```python
from build123d import *

# Parameters (mm, degrees)
SKETCH2_R               = 31.5
SKETCH2_R_2             = 4.5
BOSS_EXTRUDE2_DEPTH     = 20
CUT_EXTRUDE1_DEPTH      = 26
CUT_EXTRUDE1_DEPTH_BACK = 80
SKETCH3_W               = 10.2
SKETCH3_H               = 12.2
SKETCH2_4_R             = 4.5
BOSS_EXTRUDE3_DEPTH     = 20
SKETCH2_5_R             = 4.5
CUT_EXTRUDE2_DEPTH      = 6
SKETCH2_6_R             = 3
CUT_EXTRUDE3_DEPTH      = 20


with BuildPart() as part:
    # Sketch2 → Boss-Extrude2 (new body)
    with BuildSketch(Plane.XY):
        Circle(SKETCH2_R)
        with Locations((-17.67766953, 17.67766953)):
            Circle(SKETCH2_R_2, mode=Mode.SUBTRACT)
        with Locations((-25, 0)):
            Circle(SKETCH2_R_2, mode=Mode.SUBTRACT)
        with Locations((-17.67766953, -17.67766953)):
            Circle(SKETCH2_R_2, mode=Mode.SUBTRACT)
        with Locations((17.67766953, 17.67766953)):
            Circle(SKETCH2_R_2, mode=Mode.SUBTRACT)
        with Locations((25, 0)):
            Circle(SKETCH2_R_2, mode=Mode.SUBTRACT)
        with Locations((17.67766953, -17.67766953)):
            Circle(SKETCH2_R_2, mode=Mode.SUBTRACT)
    extrude(amount=BOSS_EXTRUDE2_DEPTH)

    # Sketch3 → Cut-Extrude1 (cut, two sides: drawn at the far end of the back side and taken through both)
    with BuildSketch(Plane(origin=(0, 32.253829663, 0), x_dir=(1, 0, 0), z_dir=(0, 1, 0)).offset(-CUT_EXTRUDE1_DEPTH_BACK)):
        with Locations((0, -9.3)):
            Rectangle(SKETCH3_W, SKETCH3_H)
    extrude(amount=CUT_EXTRUDE1_DEPTH + CUT_EXTRUDE1_DEPTH_BACK, mode=Mode.SUBTRACT)

    # Sketch2<4> → Boss-Extrude3 (add)
    with BuildSketch(Plane.XY):
        with Locations((-17.67766953, 17.67766953)):
            Circle(SKETCH2_4_R)
        with Locations((-25, 0)):
            Circle(SKETCH2_4_R)
        with Locations((-17.67766953, -17.67766953)):
            Circle(SKETCH2_4_R)
        with Locations((17.67766953, 17.67766953)):
            Circle(SKETCH2_4_R)
        with Locations((25, 0)):
            Circle(SKETCH2_4_R)
        with Locations((17.67766953, -17.67766953)):
            Circle(SKETCH2_4_R)
    extrude(amount=BOSS_EXTRUDE3_DEPTH)

    # Sketch2<5> → Cut-Extrude2 (cut)
    with BuildSketch(Plane.XY):
        with Locations((-17.67766953, 17.67766953)):
            Circle(SKETCH2_5_R)
        with Locations((-25, 0)):
            Circle(SKETCH2_5_R)
        with Locations((-17.67766953, -17.67766953)):
            Circle(SKETCH2_5_R)
        with Locations((17.67766953, 17.67766953)):
            Circle(SKETCH2_5_R)
        with Locations((25, 0)):
            Circle(SKETCH2_5_R)
        with Locations((17.67766953, -17.67766953)):
            Circle(SKETCH2_5_R)
    extrude(amount=CUT_EXTRUDE2_DEPTH, mode=Mode.SUBTRACT)

    # Sketch2<6> → Cut-Extrude3 (cut)
    with BuildSketch(Plane.XY):
        with Locations((-17.67766953, 17.67766953)):
            Circle(SKETCH2_6_R)
        with Locations((-25, 0)):
            Circle(SKETCH2_6_R)
        with Locations((-17.67766953, -17.67766953)):
            Circle(SKETCH2_6_R)
        with Locations((17.67766953, 17.67766953)):
            Circle(SKETCH2_6_R)
        with Locations((25, 0)):
            Circle(SKETCH2_6_R)
        with Locations((17.67766953, -17.67766953)):
            Circle(SKETCH2_6_R)
    extrude(amount=CUT_EXTRUDE3_DEPTH, mode=Mode.SUBTRACT)


solid = part.part
```
Model file for the job. Use its own axes, mm. A direction names the side the tool comes from. Round coordinates to 2 decimals unless told otherwise and drop trailing zeros. Loops run counter-clockwise (first coordinate to the right, second up) from the corner with the lowest first, then second, coordinate; pieces in that order, holes last. Notation, with made-up numbers: M 35.25,-11 L 77.25,-11 A23 ccw 77.25,10 Z; hole C 51,-4 d11. An arc over 180 degrees is marked long. Put each result on its own line as item: value. Start each with the question number.
Item 1: Cut at B-B (x = 0). List the corners of the cut face in (y, z).
Item 2: Cut at A-A (y = 0). List the corners of the cut face in (x, z), then the cut area to 3 significant figures.
Item 3: Cut at D-D (x = -17). List the corners of the cut face in (y, z), then the cut area to 3 significant figures.
Item 4: Drill centre lines: line 1 along Z through (x, y) = (-2, 3); line 2 along X through (y, z) = (-2.5, 5.75); line 3 along Y through (x, z) = (21, 4.75). Where is each one in solid material? Low to high.
Item 5: 3-axis set-ups, long thin cutter, end or side, ignore diameter. For faces 1 (the face through (0, 0, 0)), 2 (the face through (-18, 21, 6)), 3 (the face through (-5.1, 0, 9)): which of +Z, -Z, +X, -X, +Y, -Y reach the whole face in a straight line?
Item 6: Mould opens along Y. For faces 4 (the face through (-20.06, -19.5, 12.9)), 5 (the face through (0, 0, 3.2)) say: released by +Y, released by -Y, zero draft, split by the parting line, or undercut.
Item 7: Cut at C-C (z = 8.5). List the corners of the cut face in (x, y), then the cut area to 3 significant figures.
Item 8: Drop flat-ended pins along their axis: P1, Ø2.5, axis at x = 16, y = -19.5, coming from the -Z side; P2, Ø10, axis at x = 10.5, z = 6.5, coming from the +Y side; P3, Ø4.5, axis at x = -16.5, y = 20, coming from the -Z side; P4, Ø12, axis at y = -19, z = 10, coming from the -X side. Give the stop position or say it passes through.
Answer block:
1. outline: M -31.5,0 L 31.5,0 L 31.5,3.2 L -31.5,3.2 Z; M -31.5,15.4 L 31.5,15.4 L 31.5,20 L -31.5,20 Z
2. outline: M -31.5,0 L -29.5,0 L -29.5,6 L -28,6 L -28,20 L -31.5,20 Z; M -22,6 L -20.5,6 L -20.5,0 L 20.5,0 L 20.5,6 L 22,6 L 22,20 L -22,20 Z; M 28,6 L 29.5,6 L 29.5,0 L 31.5,0 L 31.5,20 L 28,20 Z; hole M -5.1,3.2 L 5.1,3.2 L 5.1,15.4 L -5.1,15.4 Z
2. area: 860 mm2
3. outline: M -26.52,0 L -22.13,0 L -22.13,6 L -20.6,6 L -20.6,20 L -26.52,20 Z; M -14.76,6 L -13.23,6 L -13.23,0 L 13.23,0 L 13.23,6 L 14.76,6 L 14.76,20 L -14.76,20 Z; M 20.6,6 L 22.13,6 L 22.13,0 L 26.52,0 L 26.52,20 L 20.6,20 Z
3. area: 790 mm2
4. line 1: 0 to 3.2, 15.4 to 20
4. line 2: -31.4 to -28.74, -21.26 to -5.1, 5.1 to 21.26, 28.74 to 31.4
4. line 3: -23.48 to -20.71, -14.64 to -2.06, 2.06 to 14.64, 20.71 to 23.48
5. face 1: -Z, +X, -X, +Y, -Y
5. face 2: -Z
5. face 3: +Y, -Y
6. face 4: undercut
6. face 5: zero draft
7. outline: M -5.1,-31.08 L -5.1,31.08 A31.5 ccw Z; M 5.1,-31.08 A31.5 ccw 5.1,31.08 Z; hole C -25,0 d6; hole C -17.68,-17.68 d6; hole C -17.68,17.68 d6; hole C 17.68,-17.68 d6; hole C 17.68,17.68 d6; hole C 25,0 d6
7. area: 2,310 mm2
8. P1: z = 6
8. P2: y = 31.02
8. P3: z = 0
8. P4: x = -28.69
